Geometry check sheet. Reference: the model listing, model coordinates, mm. A direction names the side the tool comes from. Round coordinates to 2 decimals unless told otherwise and drop trailing zeros. Write each loop counter-clockwise with the first axis right and the second up, starting at its lowest first coordinate (ties: lowest second). Pieces come first, ordered by that corner, then holes. Notation, with made-up numbers: M 59.5,86.25 L 68.5,86.25 A13 cw 68.5,93.25 Z; hole C 71.25,36.25 d2. An arc over 180 degrees is marked long. Use a Markdown table: item, result.
```python
from build123d import *

# Parameters (mm, degrees)
SKETCH_R      = 30
SKETCH_R_2    = 21
PAD_DEPTH     = 4
SKETCH001_R   = 25
SKETCH001_R_2 = 21
PAD001_DEPTH  = 36
SKETCH002_R   = 25
SKETCH002_R_2 = 21
PAD002_DEPTH  = 10


with BuildPart() as part:
    # Sketch → Pad (new body)
    with BuildSketch(Plane.XY):
        Circle(SKETCH_R)
        Circle(SKETCH_R_2, mode=Mode.SUBTRACT)
    extrude(amount=PAD_DEPTH)

    # Sketch001 (on Face3 of Pad) → Pad001 (join)
    with BuildSketch(Plane(origin=(0, 0, 0), x_dir=(1, 0, 0), z_dir=(0, 0, -1))):
        Circle(SKETCH001_R)
        Circle(SKETCH001_R_2, mode=Mode.SUBTRACT)
    extrude(amount=PAD001_DEPTH)

    # Sketch002 (on Face3 of Pad001) → Pad002 (join)
    with BuildSketch(Plane.XY.offset(4)):
        Circle(SKETCH002_R)
        Circle(SKETCH002_R_2, mode=Mode.SUBTRACT)
    extrude(amount=PAD002_DEPTH)


solid = part.part
```
Item 1: Go/stop test with flat-tipped pins: pin 1 (8 mm diameter, centred on y = 13, z = -26, fed in from -X); pin 2 (5 mm diameter, centred on x = 3, z = 1, fed in from +Y); pin 3 (5 mm diameter, centred on y = -23.5, z = -26, fed in from +X). Record where each tip stops, or that it passes through.
Outcome:
| item | result |
|---|---|
| pin 1 | stops at x = -23.32 |
| pin 2 | stops at y = 30 |
| pin 3 | stops at x = 13.56 |
Item 2: Mould release check, pull along Y, two halves, no side actions. Record for faces 4 (the face through (-7, 25, 0)), 5 (the face through (20.03, 6.31, -11.35)), 6 (the face through (23.846, 7.509, 8.93)): +Y half, -Y half, draft (parallel to the pull), parting line (faces both ways), or undercut.
Outcome:
| item | result |
|---|---|
| face 4 | draft |
| face 5 | undercut |
| face 6 | parting line |
Item 3: Cross-section at A-A, the plane x = 0. Record the cut outline in (y, z).
Outcome:
| item | result |
|---|---|
| outline | M -30,0 L -25,0 L -25,-36 L -21,-36 L -21,14 L -25,14 L -25,4 L -30,4 Z; M 21,-36 L 25,-36 L 25,0 L 30,0 L 30,4 L 25,4 L 25,14 L 21,14 Z |
Item 4: Access from +Z, -Z, +X, -X, +Y, -Y to the whole of each face (thin tool, end or side, straight path). Record for faces 1 (the face through (23.846, -7.509, -17.748)), 2 (the face through (-29.97, 1.32, 1.97)), 3 (the face through (-7, 25, 4)).
Outcome:
| item | result |
|---|---|
| face 1 | -Z |
| face 2 | +Z, -Z |
| face 3 | +Z |
Item 5: Material ranges on line 1 along X through (y, z) = (0, -5); line 2 along Z through (x, y) = (-24.5, 8), recorded low to high. Write a range as from..to.
Outcome:
| item | result |
|---|---|
| line 1 | x = -25..-21, 21..25 |
| line 2 | z = 0..4 |
Item 6: Cross-section at C-C, the plane z = -3. Record the cut outline in (x, y).
Outcome:
| item | result |
|---|---|
| outline | C 0,0 d50; hole C 0,0 d42 |
